Input: part model. Units: mm. Frame: model coordinates. Coordinates: 2 decimals unless noted, no trailing zeros. Loops run counter-clockwise (first coordinate to the right, second up) from the corner with the lowest first, then second, coordinate; pieces in that order, holes last.
Autodesk Inventor part; units mm, degrees
ref_plane "YZ Plane" through (0, 0, 0) normal (1, 0, 0) x (0, 1, 0)
ref_plane "XZ Plane" through (0, 0, 0) normal (0, 1, 0) x (-1, 0, 0)
ref_plane "XY Plane" through (0, 0, 0) normal (0, 0, 1) x (1, 0, 0)
sketch "Sketch1" plane through (0, 0, 0) normal (0, 0, 1) x (1, 0, 0)
  line L0 (0, 0) -> (-166.8883, 119.871)
  line L1 (-166.8883, 119.871) -> (118.9149, 119.871)
  line L2 (118.9149, 119.871) -> (118.9149, 0)
  line L3 (118.9149, 0) -> (0, 0)
  line L4 (385.7085, 119.871) -> (-223.8915, 119.871)
  line L5 (-0.2224, 6.0906) -> (-134.4097, 122.7379)
  line L6 (159.6989, 0) -> (330.9455, 0)
  line L7 (-119.1192, 85.4511) -> (-192.965, 138.6604)
extrude "Extrusion1" add sketch "Sketch1" against normal blind 5
properties part number "frontLeftSidePlateV2"
Item 1: Section query B-B (y = 9.5). Output: boundary loops of the cut face in (x, z).
Result:
outline: (-13.23, -5) - (118.91, -5) - (118.91, 0) - (-13.23, 0) - close
Item 2: Section query A-A (z = -2.2). Output: boundary loops of the cut face in (x, y).
Result:
outline: (-166.89, 119.87) - (0, 0) - (118.91, 0) - (118.91, 119.87) - close
Item 3: Line query: L1, parallel to X at y = 74.5, z = -2.25; L2, parallel to X at y = 62.5, z = -1.15; L3, parallel to Y at x = -143, z = -2.6. Output: solid intervals per line, ascending.
Result:
L1: x = -103.72 to 118.91
L2: x = -87.01 to 118.91
L3: y = 102.71 to 119.87
Item 4: Contact query for a flat-ended pin moving along its axis: P1, Ø1, axis at x = 9.5, z = -1, coming from the -Y side. Output: stop coordinate, or through.
Result:
P1: stops at y = 0
